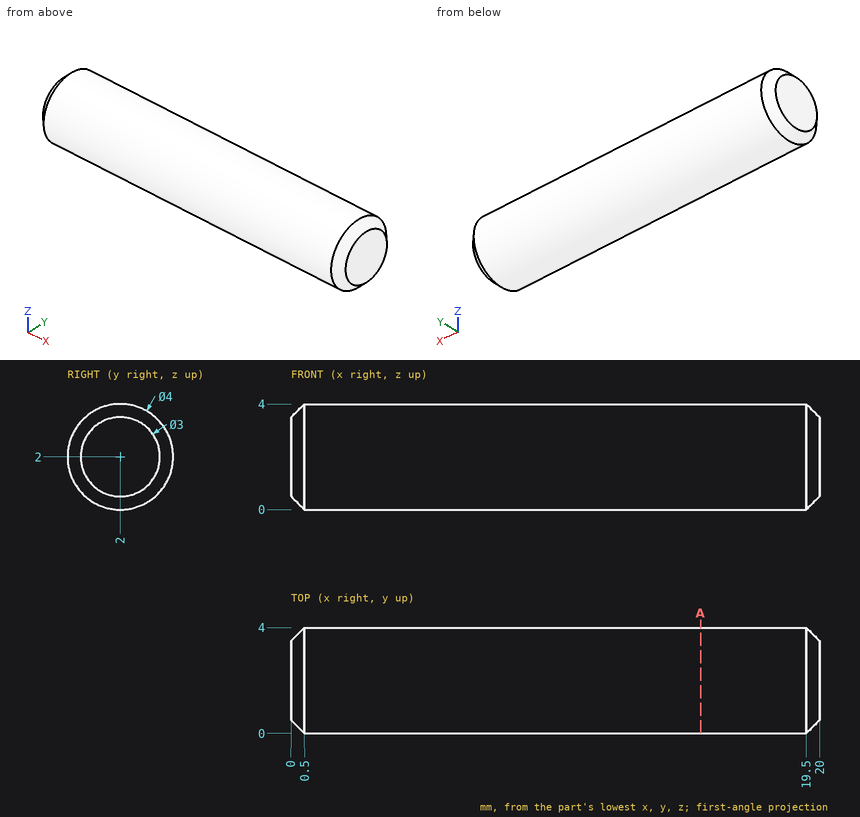
The drawing under review shows one solid part. Ordinate dimensions are in mm from its lowest x, y, z. Give positions to 0.01 mm unless a question says otherwise; leave off trailing zeros. Loops run counter-clockwise (first coordinate to the right, second up) from the corner with the lowest first, then second, coordinate; pieces in that order, holes last. Notation, with made-up numbers: M -6,14.5 L 35,14.5 A31 ccw 35,52.5 Z; hole C -36,-29 d8. An arc over 180 degrees is marked long. Return JSON: item names as keys, results as strings. Group by question number.
Item 1: We need section A-A (x = 15.5). Give the boundary of the cut face in (y, z), and give its area (3 significant figures).
Item 2: For probe 1 along Y at (x, z) = (14.25, 1.9); probe 2 along Y at (x, z) = (8, 2.5); probe 3 along Z at (x, y) = (5.25, 2.15), list the stretches that pass through material, from the lowest coordinate up.
Item 3: Insertion check: pin 1 Ø1.5 at (x, y) = (5, 1.5) entering from +Z. The pin has a flat end and moves straight along its axis. Give the tip position at first contact, or say it passes through.
Output:
{
 "1": {"outline": "C 2,2 d4", "area": "12.6 mm^2"},
 "2": {"probe 1": "y = 0 to 4", "probe 2": "y = 0.06 to 3.94", "probe 3": "z = 0.01 to 3.99"},
 "3": {"pin 1": "stops at z = 4"}
}
